Build history of the part. All positions in model axes, mm. Coordinates: 2 decimals unless noted, no trailing zeros. Write each loop counter-clockwise with the first axis right and the second up, starting at its lowest first coordinate (ties: lowest second). Pieces come first, ordered by that corner, then holes. Notation, with made-up numbers: (48, -5) -> (97, -5) arc R18 cw to (97, 18) -> close; hole circle Ø5 at (18, -34.5). An arc over 180 degrees is marked (long way). Write each question's results on one line, items separated by ' | '. Start each with the question number.
Q1. Saw through at D-D on x = 5.25. Give the cut face in (y, z), and give its area (3 significant figures).
Q2. Two-plate mould, pull along X, no slides. Class faces 1 (the face through (0, 5.08, 6)), 2 (the face through (0.29, -1.32, 6.26)): released by +X, released by -X, zero draft, split by the parting line, or undercut.
Q3. Drop flat-ended pins along their axis: pin 1 Ø2 at (x, z) = (-4, 5) entering from +Y; pin 2 Ø3 at (y, z) = (2.5, 1.5) entering from +X. Give the stop position or say it passes through.
Q4. Saw through at B-B on z = 5.5. Give the cut face in (x, y), and give its area (3 significant figures).
Q5. Saw through at C-C on x = -5. Give the cut face in (y, z), and give its area (3 significant figures).
Q6. Saw through at A-A on x = 0. Give the cut face in (y, z), and give its area (3 significant figures).
Q7. Drill centre lines: line 1 (Y direction, x = 0, z = 2.5); line 2 (X direction, y = -1, z = 5); line 3 (X direction, y = -0.5, z = 6.25). Where is each one in solid material? Low to high.
from build123d import *

# Parameters (mm, degrees)
SKETCH1_R             = 5.08
BOSS_EXTRUDE1_DEPTH   = 12.7
M3X0_5_TAPPED_HOLE1_D = 2.7


with BuildPart() as part:
    # Sketch1 → Boss-Extrude1 (new body)
    with BuildSketch(Plane.XY):
        Circle(SKETCH1_R)
        with BuildLine():
            Line((-2.932939367, 5.08), (-4.399409037, 2.540000024))
            ThreePointArc((-4.399409037, 2.540000024), (-2.539999988, 4.399409058), (0, 5.08))
            Line((0, 5.08), (-2.932939367, 5.08))
        make_face()
        with BuildLine():
            Line((2.932939367, 5.08), (0, 5.08))
            ThreePointArc((0, 5.08), (2.539999994, 4.399409055), (4.399409045, 2.540000012))
            Line((4.399409045, 2.540000012), (2.932939367, 5.08))
        make_face()
        with BuildLine():
            ThreePointArc((5.08, 0), (4.906903196, -1.314800756), (4.399409045, -2.540000012))
            Line((4.399409045, -2.540000012), (5.865878735, 0))
            Line((5.865878735, 0), (4.399409045, 2.540000012))
            ThreePointArc((4.399409045, 2.540000012), (4.906903196, 1.314800756), (5.08, 0))
        make_face()
        with BuildLine():
            ThreePointArc((4.399409045, -2.540000012), (2.539999994, -4.399409055), (0, -5.08))
            Line((0, -5.08), (2.932939367, -5.08))
            Line((2.932939367, -5.08), (4.399409045, -2.540000012))
        make_face()
        with BuildLine():
            Line((-4.399409037, 2.540000024), (-5.865878735, 0))
            Line((-5.865878735, 0), (-4.399409045, -2.540000012))
            ThreePointArc((-4.399409045, -2.540000012), (-5.08, 7e-09), (-4.399409037, 2.540000024))
        make_face()
        with BuildLine():
            ThreePointArc((0, -5.08), (-2.539999994, -4.399409055), (-4.399409045, -2.540000012))
            Line((-4.399409045, -2.540000012), (-2.932939367, -5.08))
            Line((-2.932939367, -5.08), (0, -5.08))
        make_face()
    extrude(amount=BOSS_EXTRUDE1_DEPTH)

    # M3x0.5 Tapped Hole1 (through all)
    with Locations(Plane.XY.offset(12.7)):
        with Locations((0, 0)):
            Hole(M3X0_5_TAPPED_HOLE1_D / 2)


solid = part.part
Returned:
1) outline: (-1.07, 0) -> (1.07, 0) -> (1.07, 12.7) -> (-1.07, 12.7) -> close | area: 27.1 mm2
2) face 1: zero draft | face 2: undercut
3) pin 1: stops at y = 4.96 | pin 2: stops at x = 5.29
4) outline: (-5.87, 0) -> (-2.93, -5.08) -> (2.93, -5.08) -> (5.87, 0) -> (2.93, 5.08) -> (-2.93, 5.08) -> close; hole circle Ø2.7 at (0, 0) | area: 83.7 mm2
5) outline: (-1.5, 0) -> (1.5, 0) -> (1.5, 12.7) -> (-1.5, 12.7) -> close | area: 38.1 mm2
6) outline: (-5.08, 0) -> (-1.35, 0) -> (-1.35, 12.7) -> (-5.08, 12.7) -> close; (1.35, 0) -> (5.08, 0) -> (5.08, 12.7) -> (1.35, 12.7) -> close | area: 94.7 mm2
7) line 1: y = -5.08 to -1.35, 1.35 to 5.08 | line 2: x = -5.29 to -0.91, 0.91 to 5.29 | line 3: x = -5.58 to -1.25, 1.25 to 5.58
